```python
from build123d import *

# Parameters (mm, degrees)
F1_DEPTH  = 25.4
F2_R      = 7.9375
F3_DEPTH  = 152.4
F4_R      = 127
F5_DEPTH  = 76.2
F6_R      = 7.9375
F7_DEPTH  = 241.3
F8_R      = 7.9375
F9_DEPTH  = 152.4
F10_R     = 127
F11_DEPTH = 76.2
F12_R     = 7.9375
F13_DEPTH = 241.3


with BuildPart() as f1:
    # F0 (on Right) → F1 (new body)
    with BuildSketch(Plane.YZ):
        Polygon((44.901281, 44.901281), (0, 0), (0, -63.5), (44.901281, -108.401281), (108.401281, -108.401281), (153.302561, -63.5), (153.302561, 0), (108.401281, 44.901281), align=None)
    extrude(amount=F1_DEPTH)

    # F2 (on face) → F3 (join)
    with BuildSketch(Plane.YZ.offset(25.4)):
        with Locations((76.651281, -31.75)):
            Circle(F2_R)
    extrude(amount=F3_DEPTH)

    # F4 (on face) → F5 (join)
    with BuildSketch(Plane.YZ.offset(177.8)):
        with Locations((76.651281, -31.75)):
            Circle(F4_R)
    extrude(amount=F5_DEPTH)

    # F6 (on face) → F7 (join)
    with BuildSketch(Plane.YZ.offset(254)):
        with Locations((76.651281, -31.75)):
            Circle(F6_R)
    extrude(amount=F7_DEPTH)

    # F8 (on face) → F9 (join)
    with BuildSketch(Plane(origin=(0, 0, 0), x_dir=(0, -1, 0), z_dir=(-1, 0, 0))):
        with Locations((-76.651281, -31.75)):
            Circle(F8_R)
    extrude(amount=F9_DEPTH)

    # F10 (on face) → F11 (join)
    with BuildSketch(Plane(origin=(-152.4, 0, 0), x_dir=(0, -1, 0), z_dir=(-1, 0, 0))):
        with Locations((-76.651281, -31.75)):
            Circle(F10_R)
    extrude(amount=F11_DEPTH)

    # F12 (on face) → F13 (join)
    with BuildSketch(Plane(origin=(-228.6, 0, 0), x_dir=(0, -1, 0), z_dir=(-1, 0, 0))):
        with Locations((-76.651281, -31.75)):
            Circle(F12_R)
    extrude(amount=F13_DEPTH)


solid = f1.part
```
Check sheet for the modelled part. Datum: model origin and axes. Units: mm. A direction names the side the tool comes from. Coordinates: 2 decimals unless noted, no trailing zeros. Order: outer loops, then holes, each group sorted by start corner. A loop starts at its lowest first (then second) coordinate and runs counter-clockwise, first axis right, second up. Notation, with made-up numbers: (-20.75, 41) -> (-15.75, 41) arc R13 ccw to (-15.75, 63) -> close; hole circle Ø6 at (-2, 63.25). An arc over 180 degrees is marked (long way). Write item = value, one per line. Start each with the question number.
1) Cross-section at C-C (z = -136.5). Enter the section's corners in (x, y), then the cut area to 3 significant figures.
2) Cross-section at D-D (y = -34). Enter the section's corners in (x, z), then the cut area to 3 significant figures.
3) Material ranges on L1, parallel to X at y = 26, z = -23; L2, parallel to X at y = 148.5, z = 26; L3, parallel to Z at x = -214, y = 75, recorded low to high.
4) Cross-section at A-A (z = 10). Enter the section's corners in (x, y), then the cut area to 3 significant figures.
5) Access from +Z, -Z, +X, -X, +Y, -Y to the whole of each face (thin tool, end or side, straight path). Record for faces 5 (the cylindrical face through (-347.561, 82.502, -26.385)), 6 (the cylindrical face through (100.533, 70.801, -26.385)), 7 (the flat face through (12.5, 22.1, -85.6)), 8 (the flat face through (13, 0, -31)).
6) Cross-section at B-B (y = 31). Enter the section's corners in (x, z), then the cut area to 3 significant figures.
7) Mould release check, pull along X, two halves, no side actions. Record for faces 1 (the flat face through (495.3, 77, -32)), 2 (the flat face through (13, 77, 44.901)), 3 (the flat face through (13, 153.303, -32)), 4 (the flat face through (-469.9, 77, -32)): +X half, -X half, draft (parallel to the pull), parting line (faces both ways), or undercut.
8) Go/stop test with flat-tipped pins: P1, Ø10, axis at y = 144.5, z = 44, coming from the +X side; P2, Ø7.5, axis at x = 7, y = 62, coming from the +Z side; P3, Ø20.5, axis at x = 17.5, z = -19, coming from the -Y side; P4, Ø10, axis at x = -91.5, y = 90, coming from the +Z side. Record where each tip stops, or that it passes through.
Ans:
q1.outline = (-228.6, 4.84) -> (-152.4, 4.84) -> (-152.4, 148.46) -> (-228.6, 148.46) -> close; (177.8, 4.84) -> (254, 4.84) -> (254, 148.46) -> (177.8, 148.46) -> close
q1.area = 21,900 mm²
q2.outline = (-228.6, -94.08) -> (-152.4, -94.08) -> (-152.4, 30.58) -> (-228.6, 30.58) -> close; (177.8, -94.08) -> (254, -94.08) -> (254, 30.58) -> (177.8, 30.58) -> close
q2.area = 19,000 mm²
q3.L1 = -228.6 to -152.4, 0 to 25.4, 177.8 to 254
q3.L2 = -228.6 to -152.4, 177.8 to 254
q3.L3 = -158.74 to 95.24
q4.outline = (-228.6, -43.29) -> (-152.4, -43.29) -> (-152.4, 196.59) -> (-228.6, 196.59) -> close; (0, 10) -> (25.4, 10) -> (25.4, 143.3) -> (0, 143.3) -> close; (177.8, -43.29) -> (254, -43.29) -> (254, 196.59) -> (177.8, 196.59) -> close
q4.area = 39,900 mm²
q5.face_5 = -X
q5.face_6 = none
q5.face_7 = -Z, -Y
q5.face_8 = +Z, -Z, -Y
q6.outline = (-228.6, -150.26) -> (-152.4, -150.26) -> (-152.4, 86.76) -> (-228.6, 86.76) -> close; (0, -94.5) -> (25.4, -94.5) -> (25.4, 31) -> (0, 31) -> close; (177.8, -150.26) -> (254, -150.26) -> (254, 86.76) -> (177.8, 86.76) -> close
q6.area = 39,300 mm²
q7.face_1 = +X half
q7.face_2 = undercut
q7.face_3 = undercut
q7.face_4 = -X half
q8.P1 = 254
q8.P2 = 44.9
q8.P3 = 0
q8.P4 = through
